```python
from build123d import *

# Parameters (mm, degrees)
BOSS_EXTRUDE1_DEPTH = 4
SKETCH2_R           = 2
CUT_EXTRUDE1_DEPTH  = 4
SKETCH3_R           = 1.5
CUT_EXTRUDE2_DEPTH  = 4
CUT_EXTRUDE3_DEPTH  = 4
SKETCH5_R           = 2
CUT_EXTRUDE4_DEPTH  = 4
SKETCH6_R           = 3.5
SKETCH6_W           = 20
SKETCH6_H           = 20
CUT_EXTRUDE5_DEPTH  = 4
CUT_EXTRUDE6_DEPTH  = 4
SKETCH9_R           = 17.5
CUT_EXTRUDE7_DEPTH  = 4
FILLET1_R           = 2


with BuildPart() as part:
    # Sketch1 → Boss-Extrude1 (new body)
    with BuildSketch(Plane(origin=(0, 0, 0), x_dir=(1, 0, 0), z_dir=(0, 1, 0))):
        with BuildLine():
            Line((0, 0), (0, -150))
            Line((0, -150), (129.903810568, -225))
            Line((129.903810568, -225), (150.403810568, -189.492958445))
            Line((150.403810568, -189.492958445), (190.024472791, -212.367958445))
            ThreePointArc((190.024472791, -212.367958445), (173.202037288, -50.001757147), (41, 45.75))
            Line((41, 45.75), (41, 0))
            Line((41, 0), (0, 0))
        make_face()
    extrude(amount=BOSS_EXTRUDE1_DEPTH)

    # Sketch2 → Cut-Extrude1 (cut)
    with BuildSketch(Plane(origin=(0, 4, 0), x_dir=(1, 0, 0), z_dir=(0, 1, 0))):
        with Locations(Location((20, -14, 0), (0, 0, 270))):
            Circle(SKETCH2_R)
        with Locations(Location((20, -55, 0), (0, 0, 270))):
            Circle(SKETCH2_R)
    extrude(amount=-CUT_EXTRUDE1_DEPTH, mode=Mode.SUBTRACT)

    # Sketch3 → Cut-Extrude2 (cut)
    with BuildSketch(Plane(origin=(0, 4, 0), x_dir=(1, 0, 0), z_dir=(0, 1, 0))):
        with Locations(Location((143.756051904, -79.992785793, 0), (0, 0, 270))):
            Circle(SKETCH3_R)
        with Locations(Location((132.506051904, -60.507214207, 0), (0, 0, 270))):
            Circle(SKETCH3_R)
        with Locations(Location((47.194219382, -135.742785793, 0), (0, 0, 270))):
            Circle(SKETCH3_R)
        with Locations(Location((35.944219382, -116.257214207, 0), (0, 0, 270))):
            Circle(SKETCH3_R)
    extrude(amount=-CUT_EXTRUDE2_DEPTH, mode=Mode.SUBTRACT)

    # Sketch4 → Cut-Extrude3 (cut)
    with BuildSketch(Plane(origin=(0, 4, 0), x_dir=(1, 0, 0), z_dir=(0, 1, 0))):
        with BuildLine():
            Line((0, -81), (0, -95))
            Line((0, -95), (60, -95))
            ThreePointArc((60, -95), (67, -88), (60, -81))
            Line((60, -81), (0, -81))
        make_face()
    extrude(amount=-CUT_EXTRUDE3_DEPTH, mode=Mode.SUBTRACT)

    # Sketch5 → Cut-Extrude4 (cut)
    with BuildSketch(Plane(origin=(0, 4, 0), x_dir=(1, 0, 0), z_dir=(0, 1, 0))):
        with Locations(Location((127.779454915, -200.679491924, 0), (0, 0, 270))):
            Circle(SKETCH5_R)
        with Locations(Location((92.27241336, -180.179491924, 0), (0, 0, 270))):
            Circle(SKETCH5_R)
    extrude(amount=-CUT_EXTRUDE4_DEPTH, mode=Mode.SUBTRACT)

    # Sketch6 → Cut-Extrude5 (cut)
    with BuildSketch(Plane(origin=(0, 4, 0), x_dir=(1, 0, 0), z_dir=(0, 1, 0))):
        with Locations(Location((155, -174, 0), (0, 0, 270))):
            Circle(SKETCH6_R)
        with Locations(Location((155, -126, 0), (0, 0, 90))):
            Circle(SKETCH6_R)
        with Locations((155, -150)):
            Rectangle(SKETCH6_W, SKETCH6_H)
        with BuildLine():
            Line((127, -146.5), (135, -146.5))
            ThreePointArc((135, -146.5), (138.5, -150), (135, -153.5))
            Line((135, -153.5), (127, -153.5))
            ThreePointArc((127, -153.5), (123.5, -150), (127, -146.5))
        make_face()
        with BuildLine():
            Line((183, -146.5), (175, -146.5))
            ThreePointArc((175, -146.5), (171.5, -150), (175, -153.5))
            Line((175, -153.5), (183, -153.5))
            ThreePointArc((183, -153.5), (186.5, -150), (183, -146.5))
        make_face()
    extrude(amount=-CUT_EXTRUDE5_DEPTH, mode=Mode.SUBTRACT)

    # Sketch8 → Cut-Extrude6 (cut)
    with BuildSketch(Plane(origin=(0, 4, 0), x_dir=(1, 0, 0), z_dir=(0, 1, 0))):
        with BuildLine():
            Line((47.631397208, -177.5), (59.755752861, -184.5))
            Line((59.755752861, -184.5), (89.755752861, -132.538475773))
            ThreePointArc((89.755752861, -132.538475773), (87.193575035, -122.976297946), (77.631397208, -125.538475773))
            Line((77.631397208, -125.538475773), (47.631397208, -177.5))
        make_face()
    extrude(amount=-CUT_EXTRUDE6_DEPTH, mode=Mode.SUBTRACT)

    # Sketch9 → Cut-Extrude7 (cut)
    with BuildSketch(Plane(origin=(0, 4, 0), x_dir=(1, 0, 0), z_dir=(0, 1, 0))):
        with Locations((0, -150)):
            Circle(SKETCH9_R)
    extrude(amount=-CUT_EXTRUDE7_DEPTH, mode=Mode.SUBTRACT)

    # Fillet1
    fillet1_edges = [part.edges().sort_by_distance(p)[0] for p in [
        (165, 2, 160),
        (165, 2, 140),
        (145, 2, 140),
        (145, 2, 160),
        (41, 2, 0),
        (41, 2, -45.75),
        (190.024472791, 2, 212.367958445),
        (150.403810568, 2, 189.492958445),
    ]]
    fillet(fillet1_edges, radius=FILLET1_R)


solid = part.part
```
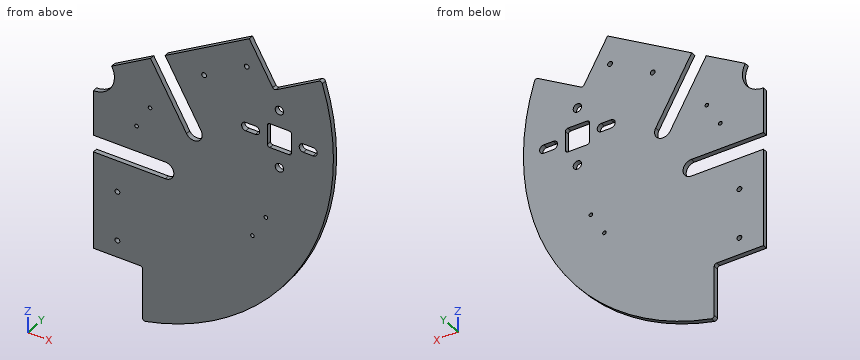
Here's how the part is built. I have some questions about the finished solid (model axes, mm). Give positions to 0.01 mm unless a question says otherwise; leave off trailing zeros. Loops run counter-clockwise (first coordinate to the right, second up) from the corner with the lowest first, then second, coordinate; pieces in that order, holes last. Notation, with made-up numbers: M 30,-19.75 L 48,-19.75 A34 cw 48,18.25 Z; hole C 15,8 d2. An arc over 180 degrees is marked long. Return JSON: item names as keys, results as strings.
Item 1: Imagine slicing it at D-D on x = 97. List the corners of the cut face in (y, z) for me.
A:
{"outline": "M 0,-24.9 L 4,-24.9 L 4,206 L 0,206 Z"}
Item 2: Imagine slicing it at A-A on z = 150. List the corners of the cut face in (x, y) for me, then the cut area to 3 significant figures.
A:
{"outline": "M 17.5,0 L 63.51,0 L 63.51,4 L 17.5,4 Z; M 79.67,0 L 123.5,0 L 123.5,4 L 79.67,4 Z; M 138.5,0 L 145,0 L 145,4 L 138.5,4 Z; M 165,0 L 171.5,0 L 171.5,4 L 165,4 Z; M 186.5,0 L 200,0 L 200,4 L 186.5,4 Z", "area": "465 mm^2"}
Item 3: Please list where these lines run through material, in increasing order: line 1 (X direction, y = 2.95, z = 152); line 2 (Z direction, x = 35, y = 2.9); line 3 (Z direction, x = 174.5, y = 0.5).
A:
{"line 1": "x = 17.39 to 62.35, 78.52 to 124.13, 137.87 to 145, 165 to 172.13, 185.87 to 199.99", "line 2": "z = 0 to 81, 95 to 115.09, 117.42 to 170.21", "line 3": "z = 52.28 to 146.54, 153.46 to 203.4"}
Item 4: I'm going to push flat-ended pins straight in: pin 1 Ø2 at (x, y) = (136.5, 0.5) entering from -Z; pin 2 Ø2 at (y, z) = (3, 90) entering from -X. Where does each tip first touch, or does it pass through?
A:
{"pin 1": "stops at z = 2.9", "pin 2": "stops at x = 66.32"}
Item 5: Imagine slicing it at C-C on y = 0.8. State how many separate pieces and enclosed holes the cut face has, then the cut area to 3 significant figures.
A:
{"separate pieces": "1", "enclosed holes": "13", "area": "35,000 mm^2"}
Item 6: Imagine slicing it at B-B on x = 53.5. List the corners of the cut face in (y, z) for me, then the cut area to 3 significant figures.
A:
{"outline": "M 0,-42.71 L 4,-42.71 L 4,81 L 0,81 Z; M 0,95 L 4,95 L 4,167.34 L 0,167.34 Z", "area": "784 mm^2"}
